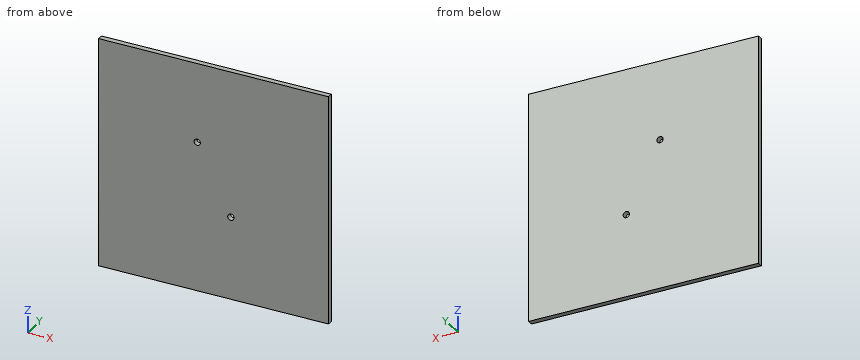
```python
from build123d import *

# Parameters (mm, degrees)
SKETCH1_W             = 101.6
SKETCH1_H             = 101.6
BOSS_EXTRUDE1_DEPTH   = 2.38125
F_2_5MM_DOWEL_HOLE1_D = 2.794


with BuildPart() as part:
    # Sketch1 → Boss-Extrude1 (new body)
    with BuildSketch(Plane.XZ.offset(-61.790986141)):
        Rectangle(SKETCH1_W, SKETCH1_H)
    extrude(amount=BOSS_EXTRUDE1_DEPTH)

    # Ø2.5mm Dowel Hole1 (through all)
    with Locations(Plane(origin=(0, 59.409736141, 0), x_dir=(-1, 0, 0), z_dir=(0, -1, 0))):
        with Locations((7.25, -15.6), (-7.65, 14.1)):
            Hole(F_2_5MM_DOWEL_HOLE1_D / 2)


solid = part.part
```
CAD build for the part. Positions are in the model's coordinates, mm. Coordinates: 2 decimals unless noted, no trailing zeros. Order: outer loops, then holes, each group sorted by start corner. A loop starts at its lowest first (then second) coordinate and runs counter-clockwise, first axis right, second up.
(1) Saw through at B-B, the plane z = -14.1. Write the cut outline in (x, y).
Solution:
outline: (-50.8, 59.41) - (6.25, 59.41) - (6.25, 61.79) - (-50.8, 61.79) - close; (9.05, 59.41) - (50.8, 59.41) - (50.8, 61.79) - (9.05, 61.79) - close
(2) Drill centre lines: L1, parallel to X at y = 60.95, z = 15.6; L2, parallel to Z at x = 7.65, y = 60.65; L3, parallel to X at y = 60.2, z = -14.1. Where is each one in solid material? Low to high.
Solution:
L1: x = -50.8 to -8.65, -5.85 to 50.8
L2: z = -50.8 to -15.5, -12.7 to 50.8
L3: x = -50.8 to 6.25, 9.05 to 50.8
(3) Saw through at A-A, the plane x = 7.65. Write the cut outline in (y, z), and give its area (3 significant figures).
Solution:
outline: (59.41, -50.8) - (61.79, -50.8) - (61.79, -15.5) - (59.41, -15.5) - close; (59.41, -12.7) - (61.79, -12.7) - (61.79, 50.8) - (59.41, 50.8) - close
area: 235 mm2
